Answer from the drawing. Dimensions are ordinates in mm from the lowest x, y and z of the part. Give positions to 0.01 mm unless a question says otherwise; leave off trailing zeros. Order: outer loops, then holes, each group sorted by start corner. A loop starts at its lowest first (then second) coordinate and runs counter-clockwise, first axis right, second up. Notation, with made-up numbers: (72.5, 22) - (102.5, 22) arc R34 ccw to (102.5, 53) - close; hole circle Ø5 at (29, -29). An arc over 180 degrees is marked (long way). Answer in a Markdown table with one row per item. Add a question column.
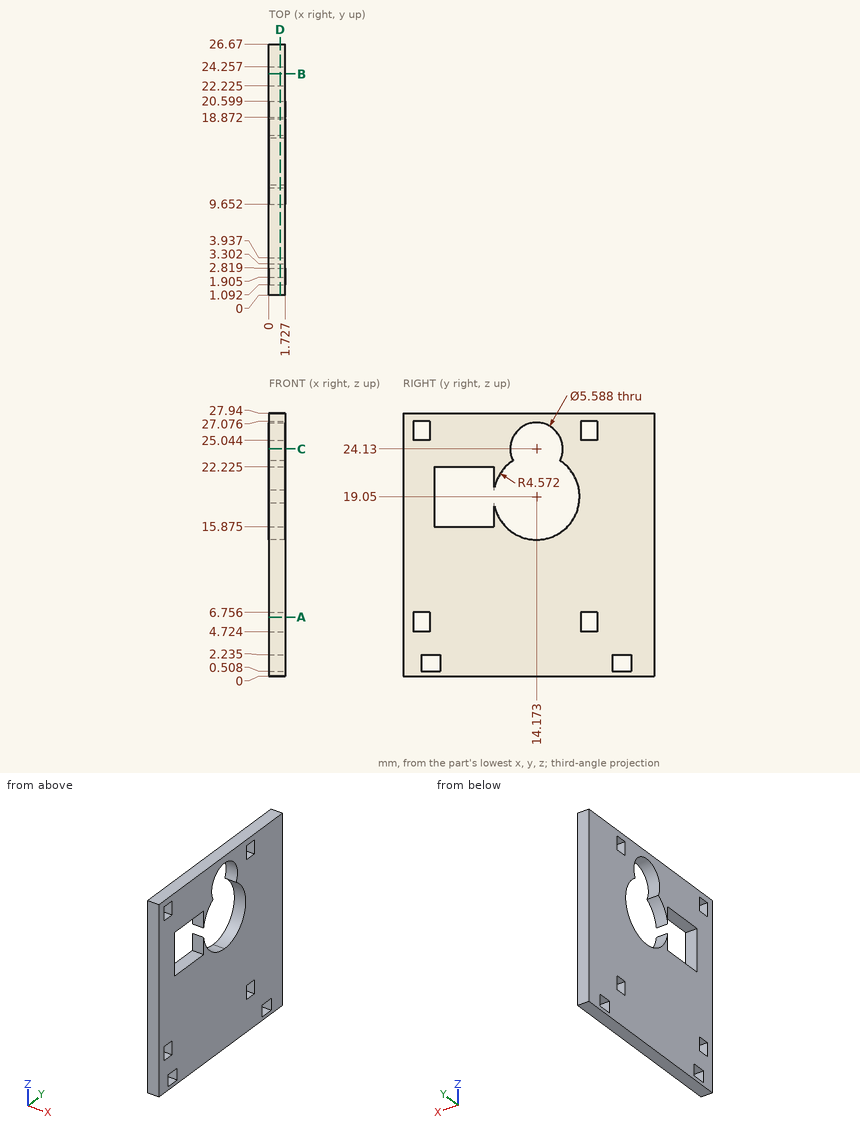
(1) This flat-tipped pin is pushed along its axis until it touches: P1, Ø4.5, axis at y = 14.17, z = 24.13, coming from the +X side. Where does it stop, or does it pass through?
(2) Find section C-C, the plane z = 24.13. Write down the section's boundary in (x, y).
(3) Find section D-D, the plane x = 1.2. Give the number of separate pieces and of enclosed holes in the cut face.
(4) Find section B-B, the plane y = 23.5. Write down the section's boundary in (x, z) (1 decimal).
(5) Find section A-A, the plane z = 6.25. Write down the section's boundary in (x, y).
(6) Straight lines are drawn through the part: line 1 (Z direction, x = 0.2, y = 3.75) (1 decimal); line 2 (Y direction, x = 0.6, z = 24.13); line 3 (Y direction, x = 0.6, z = 26.25) (1 decimal). For each, find the intervals that lie inside material, in ascending order.
Answer key:
| question | item | result |
|---|---|---|
| 1 | P1 | through |
| 2 | outline | (0, 0) - (1.73, 0) - (1.73, 11.38) - (0, 11.38) - close; (0, 16.97) - (1.73, 16.97) - (1.73, 26.67) - (0, 26.67) - close |
| 3 | separate pieces | 1 |
| 3 | enclosed holes | 7 |
| 4 | outline | (0, 0) - (1.7, 0) - (1.7, 0.5) - (0, 0.5) - close; (0, 2.2) - (1.7, 2.2) - (1.7, 27.9) - (0, 27.9) - close |
| 5 | outline | (0, 0) - (1.73, 0) - (1.73, 1.09) - (0, 1.09) - close; (0, 2.82) - (1.73, 2.82) - (1.73, 18.87) - (0, 18.87) - close; (0, 20.6) - (1.73, 20.6) - (1.73, 26.67) - (0, 26.67) - close |
| 6 | line 1 | 0 to 0.5, 2.2 to 15.9, 22.2 to 27.9 |
| 6 | line 2 | 0 to 11.38, 16.97 to 26.67 |
| 6 | line 3 | 0 to 1.1, 2.8 to 12.4, 16 to 18.9, 20.6 to 26.7 |
